The model under review builds one solid part; all positions refer to its coordinate system, in mm. Round coordinates to 2 decimals unless told otherwise and drop trailing zeros. Order: outer loops, then holes, each group sorted by start corner. A loop starts at its lowest first (then second) coordinate and runs counter-clockwise, first axis right, second up. Notation, with made-up numbers: M 69.25,25.5 L 78.25,25.5 A15 ccw 78.25,54.5 Z; hole C 28,74 d1. An arc over 180 degrees is marked long. Use a Markdown table: item, result. Add a question column.
1. Insertion check: P1, Ø0.6, axis at x = -101, z = 2, coming from the -Y side; P2, Ø1.5, axis at y = 16.5, z = 1.5, coming from the +X side (3 decimals); P3, Ø1, axis at y = 22, z = 2, coming from the -X side (3 decimals). Each pin has a flat end and moves straight along its axis. Give the tip position at first contact, or say it passes through.
2. Consider section B-B on x = -50.8. State the section outline as (y, z) points (3 decimals).
3. Consider section A-A on y = 19.05. State the section outline as (x, z) points (3 decimals).
4. Consider section D-D on y = 88.9. State the section outline as (x, z) points (3 decimals), then the cut area to 3 significant figures.
5. Consider section C-C on z = 2.55. Count the separate pieces of the cut face and the enclosed holes in it, then the cut area to 3 significant figures.
6. To check wall thickness, follow probe 1 along Y at (x, z) = (-25.4, 1.1); probe 2 along Y at (x, z) = (-26, 0.8); probe 3 along X at (y, z) = (5, 2.5). State the ranges of each line that lie inside material, in increasing order.
Autodesk Inventor part; units mm, degrees
ref_plane "YZ Plane" through (0, 0, 0) normal (1, 0, 0) x (0, 1, 0)
ref_plane "XZ Plane" through (0, 0, 0) normal (0, 1, 0) x (-1, 0, 0)
ref_plane "XY Plane" through (0, 0, 0) normal (0, 0, 1) x (1, 0, 0)
sketch "Sketch1" plane through (0, 0, 0) normal (0, 0, 1) x (1, 0, 0)
  line L0 (0, 0) -> (-101.6, 0)
  line L1 (-101.6, 0) -> (-101.6, 101.6)
  line L2 (-95.25, 101.6) -> (0, 101.6)
  circle A0 centre (-76.2, 88.9) radius 2.5797
  circle A1 centre (-76.2, 63.5) radius 2.5797
  circle A2 centre (-25.4, 88.9) radius 2.5797
  circle A3 centre (-25.4, 63.5) radius 2.5797
  circle A4 centre (-50.8, 19.05) radius 9.525
  circle A5 centre (-76.2, 31.75) radius 2.5797
  circle A6 centre (-76.2, 6.35) radius 2.5797
  circle A7 centre (-25.4, 31.75) radius 2.5797
  circle A8 centre (-25.4, 6.35) radius 2.5797
  line L3 (-22.225, 0) -> (-79.375, 0)
  line L4 (-101.6, 50.677) -> (-101.6, 95.25)
  line L5 (-101.6, 101.6) -> (-6.35, 101.6)
  line L6 (0, 0) -> (-15.875, 0)
  line L7 (-15.875, 6.35) -> (-15.875, 31.873)
  line L8 (-101.6, 0) -> (-85.725, 0)
  line L9 (-85.725, 6.35) -> (-85.725, 31.873)
  line L10 (-85.725, 47.625) -> (-101.6, 47.625)
  line L11 (-101.6, 47.625) -> (-101.6, 0)
  line L12 (-101.6, 47.625) -> (-88.8573, 47.625)
  line L13 (-101.6, 26.0622) -> (-101.6, 47.625)
  line L14 (0, 95.25) -> (0, 50.677)
  line L15 (-15.875, 47.625) -> (0, 47.625)
  line L16 (-15.875, 47.625) -> (0, 47.625)
  line L17 (0, 47.625) -> (0, 34.925)
  line L18 (0, 34.925) -> (-15.875, 34.925)
  line L19 (-15.875, 34.925) -> (-15.875, 47.625)
  line L20 (-85.725, 47.625) -> (-101.6, 47.625)
  line L21 (-101.6, 47.625) -> (-101.6, 34.925)
  line L22 (-101.6, 34.925) -> (-85.725, 34.925)
  line L23 (-85.725, 34.925) -> (-85.725, 47.625)
  line L24 (-101.6, 41.275) -> (-85.725, 41.275)
  line L25 (-13.4918, 36.8315) -> (-2.3832, 45.7185)
  line L26 (-88.1082, 36.8315) -> (-99.2168, 45.7185)
  arc A9 (-101.6, 50.677) -> (-99.2168, 45.7185) centre (-95.25, 50.677) ccw
  arc A10 (-85.725, 31.873) -> (-88.1082, 36.8315) centre (-92.075, 31.873) ccw
  arc A11 (-2.3832, 45.7185) -> (0, 50.677) centre (-6.35, 50.677) ccw
  arc A12 (-13.4918, 36.8315) -> (-15.875, 31.873) centre (-9.525, 31.873) ccw
  arc A13 (-22.225, 0) -> (-15.875, 6.35) centre (-22.225, 6.35) ccw
  arc A14 (-85.725, 6.35) -> (-79.375, 0) centre (-79.375, 6.35) ccw
  arc A15 (0, 95.25) -> (-6.35, 101.6) centre (-6.35, 95.25) ccw
  arc A16 (-95.25, 101.6) -> (-101.6, 95.25) centre (-95.25, 95.25) ccw
  point P0 (0, 101.6)
  point P1 (0, 88.9)
  point P2 (-100.8185, 47.625)
  point P3 (-6.35, 101.6)
  point P4 (-101.6, 95.25)
  point P5 (-95.25, 101.6)
  dimension "d0" = 101.6
  dimension "d1" = 101.6
  dimension "d4" = 25.4
  dimension "d7" = 50.8
  dimension "d10" = 12.7
  dimension "d11" = 25.4
  dimension "d12" = 5.1594
  dimension "d13" = 19.05
  dimension "d14" = 5.1594
  dimension "d17" = 25.4
  dimension "d20" = 50.8
  dimension "d23" = 25.4
  dimension "d24" = 6.35
  dimension "d26" = 50.8
  dimension "d29" = 12.7
  dimension "d30" = 101.6
  dimension "d31" = 101.6
  dimension "d32" = 15.875
  dimension "d34" = 101.6
  dimension "d35" = 12.7
  dimension "d36" = 41.275
  dimension "d37" = 6.35
  dimension "d38" = 6.35
  dimension "d39" = 6.35
  dimension "d40" = 88.8572
  dimension "d41" = 21.5628
  dimension "d42" = 6.35
extrude "Extrusion1" add sketch "Sketch1" along normal blind 3.175 contours L0 A14 L9 A10 L22 L23 L10 A9 L1 A16 L2 A15 L14 A11 L15 L19 L18 A12 L7 A13 | L18 L19 L15 A11 L25 A12 | A10 L26 L24 L23 L22 | L24 L26 A9 L10 L23 | L1 A9 L10
properties part number "Dipper Plate"
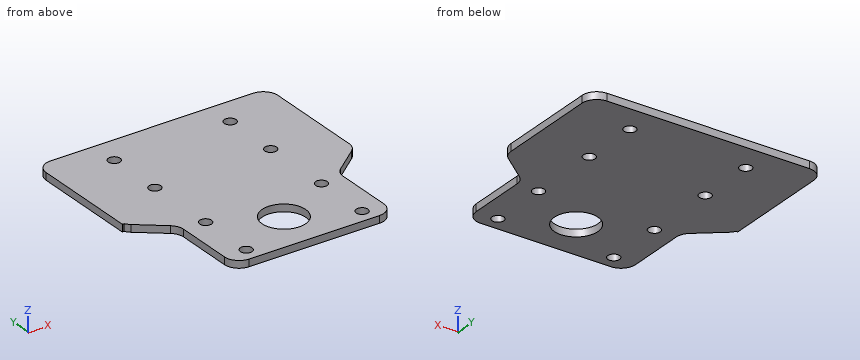
Answer block:
| question | item | result |
|---|---|---|
| 1 | P1 | y = 47.42 |
| 1 | P2 | x = -15.875 |
| 1 | P3 | x = -85.725 |
| 2 | outline | M 0,0 L 9.525,0 L 9.525,3.175 L 0,3.175 Z; M 28.575,0 L 101.6,0 L 101.6,3.175 L 28.575,3.175 Z |
| 3 | outline | M -85.725,0 L -60.325,0 L -60.325,3.175 L -85.725,3.175 Z; M -41.275,0 L -15.875,0 L -15.875,3.175 L -41.275,3.175 Z |
| 4 | outline | M -101.6,0 L -78.78,0 L -78.78,3.175 L -101.6,3.175 Z; M -73.62,0 L -27.98,0 L -27.98,3.175 L -73.62,3.175 Z; M -22.82,0 L 0,0 L 0,3.175 L -22.82,3.175 Z |
| 4 | area | 290 mm^2 |
| 5 | separate pieces | 1 |
| 5 | enclosed holes | 9 |
| 5 | area | 8,530 mm^2 |
| 6 | probe 1 | 0 to 3.77, 8.93 to 29.17, 34.33 to 60.92, 66.08 to 86.32, 91.48 to 101.6 |
| 6 | probe 2 | 0 to 3.84, 8.86 to 29.24, 34.26 to 60.99, 66.01 to 86.39, 91.41 to 101.6 |
| 6 | probe 3 | -85.58 to -78.4, -74 to -27.6, -23.2 to -16.02 |
